Could you check a few things on this model? Use its own coordinates, in mm. Face numbers are marked on the shaded views. A direction names the side the tool comes from. Give positions to 0.01 mm unless a question says otherwise; leave off trailing zeros. Order: outer loops, then holes, each group sorted by start corner. A loop starts at its lowest first (then second) coordinate and runs counter-clockwise, first axis right, second up.
from build123d import *

# Parameters (mm, degrees)
F1_DEPTH = 25
F2_DEPTH = 20
F3_R     = 3.843017
F4_DEPTH = 25
F5_R     = 6.951677
F5_R_2   = 4
F6_DEPTH = 10


with BuildPart() as f1:
    # F0 (on Top) → F1 (new body)
    with BuildSketch(Plane.XY):
        Polygon((14.980248, -13.11259), (2.429798, -2.581512), (-0.571601, -9.866924), (13.009035, -15.46179), align=None)
        Polygon((2.429798, -2.581512), (-13.757027, 11.000847), (-37.870464, -17.736428), (-9.133189, -41.849865), (13.009035, -15.46179), (-0.571601, -9.866924), align=None)
    extrude(amount=F1_DEPTH)

    # F0 (on Top) → F2 (join)
    with BuildSketch(Plane.XY):
        Polygon((13.717991, 24.818756), (2.429798, -2.581512), (14.980248, -13.11259), (13.009035, -15.46179), (34.114079, -24.156516), (48.403671, 10.529164), align=None)
    extrude(amount=F2_DEPTH)

    # F3 (on Top) → F4 (cut)
    with BuildSketch(Plane.XY):
        with Locations((-15.104588, -2.620658)):
            Circle(F3_R)
        with Locations((-25.983153, -14.315117)):
            Circle(F3_R)
        with Locations((-6.129771, -9.011817)):
            Circle(F3_R)
        with Locations((-17.008336, -20.706276)):
            Circle(F3_R)
        with Locations((2.437101, -15.810922)):
            Circle(F3_R)
        with Locations((-8.441464, -27.50538)):
            Circle(F3_R)
        with Locations((17.939058, 13.017283)):
            Circle(F3_R)
        with Locations((22.834416, 1.050857)):
            Circle(F3_R)
        with Locations((28.273696, -10.507619)):
            Circle(F3_R)
    extrude(amount=F4_DEPTH, mode=Mode.SUBTRACT)

    # F5 (on Top) → F6 (join)
    with BuildSketch(Plane.XY):
        with Locations((1.257815, 1.869077)):
            Circle(F5_R)
        with Locations((1.257815, 1.869077)):
            Circle(F5_R_2, mode=Mode.SUBTRACT)
    extrude(amount=F6_DEPTH)


solid = f1.part
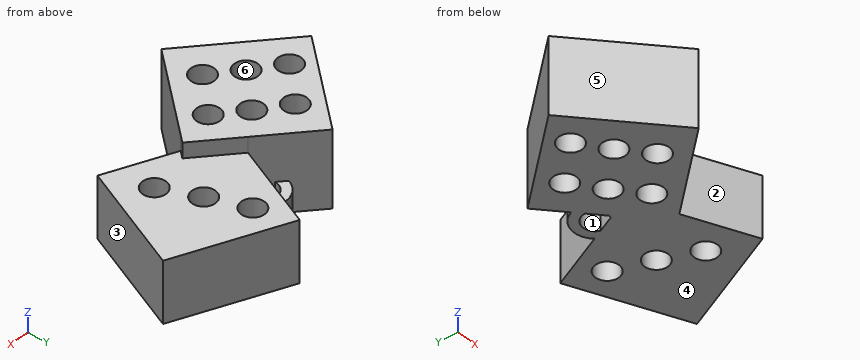
Item 1: Imagine slicing it at D-D on z = 12.5. Give the number of separate pieces and of enclosed holes in the cut face, then the cut area to 3 significant figures.
Findings:
separate pieces: 1
enclosed holes: 9
area: 2,310 mm2
Item 2: Imagine slicing it at B-B on x = 31. List the corners of the cut face in (y, z) for me, then the cut area to 3 significant figures.
Findings:
outline: (-22.87, 0) - (-13.22, 0) - (-13.22, 20) - (-22.87, 20) - close; (-7.8, 0) - (17.7, 0) - (17.7, 20) - (-7.8, 20) - close
area: 703 mm2
Item 3: Imagine slicing it at C-C on z = 22.75. List the corners of the cut face in (x, y) for me, then the cut area to 3 significant figures.
Findings:
outline: (-37.87, -17.74) - (-9.13, -41.85) - (14.98, -13.11) - (-13.76, 11) - close; hole circle Ø7.69 at (-25.98, -14.32); hole circle Ø7.69 at (-17.01, -20.71); hole circle Ø7.69 at (-15.1, -2.62); hole circle Ø7.69 at (-8.44, -27.51); hole circle Ø7.69 at (-6.13, -9.01); hole circle Ø7.69 at (2.44, -15.81)
area: 1,130 mm2
Item 4: Imagine slicing it at A-A on x = 20.5. List the corners of the cut face in (y, z) for me, then the cut area to 3 significant figures.
Findings:
outline: (-18.55, 0) - (-2, 0) - (-2, 20) - (-18.55, 20) - close; (4.1, 0) - (10.15, 0) - (10.15, 20) - (4.1, 20) - close; (15.88, 0) - (22.02, 0) - (22.02, 20) - (15.88, 20) - close
area: 575 mm2
Item 5: For the marked faces 1, 2 and 3, which set-ups out of +Z, -Z, +X, -X, +Y, -Y let a thin tool reach every point of the face, with its end or its side?
Findings:
face 1: +Z, -Z
face 2: +Z, -Z, -Y
face 3: +Z, -Z, +X, -Y
Item 6: For pin 1 (0.8 mm diameter, centred on x = 2, y = -2, fed in from +Z); pin 2 (6 mm diameter, centred on x = 17.94, y = 13.02, fed in from -Z); pin 3 (2 mm diameter, centred on y = 4, z = 12.5, fed in from +X); pin 4 (12 mm diameter, centred on y = 4.5, z = 3.5, fed in from -X), each with a flat end and sliding along its axis, tell me the tip position at first contact or that it passes through.
Findings:
pin 1: stops at z = 25
pin 2: passes through
pin 3: stops at x = 46.13
pin 4: stops at x = -24.25
Item 7: We'd pull the mould along X, two halves only. Please class the marked faces 4, 5 and 6: +X half, -X half, draft (parallel to the pull), parting line (faces both ways), or undercut.
Findings:
face 4: draft
face 5: -X half
face 6: undercut
Item 8: Please list where these lines run through material, in increasing order: line 1 along X through (y, z) = (4, 17); line 2 along X through (y, z) = (-6, 8); line 3 along X through (y, z) = (-14, 18).
Findings:
line 1: x = -19.63 to -5.41, 5.14 to 20.37, 25.3 to 45.71
line 2: x = -28.02 to -16.93, -13.27 to -8.52, -3.74 to 41.59
line 3: x = -34.74 to -29.81, -22.15 to -0.95, 5.83 to 26.67, 29.88 to 38.3
